```python
from build123d import *

# Parameters (mm, degrees)
BASESTEELANGLE_DEPTH = 150
TOEFILLET_R          = 10


with BuildPart() as part:
    # Sketch1 → BaseSteelAngle (new, symmetric)
    with BuildSketch(Plane.XY):
        with BuildLine():
            Line((0, 100), (0, 0))
            Line((0, 0), (100, 0))
            Line((100, 0), (100, 10))
            Line((100, 10), (22, 10))
            ThreePointArc((22, 10), (13.514718626, 13.514718626), (10, 22))
            Line((10, 22), (10, 100))
            Line((10, 100), (0, 100))
        make_face()
    extrude(amount=BASESTEELANGLE_DEPTH, both=True)

    # ToeFillet
    toefillet_edges = [part.edges().sort_by_distance(p)[0] for p in [
        (10, 100, 0),
        (100, 10, 0),
    ]]
    fillet(toefillet_edges, radius=TOEFILLET_R - 0.0001)  # a hair under: the kernel refuses the full size


solid = part.part
```
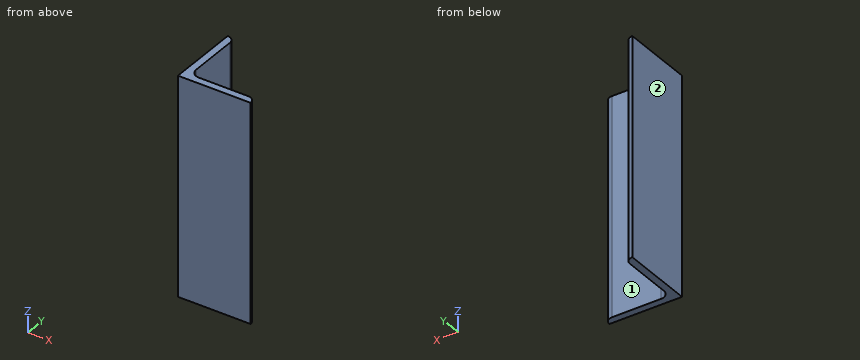
For this review, take the finished solid that the model builds, in its own axes (mm). Face numbers are marked on the shaded views. A direction names the side the tool comes from. Coordinates: 2 decimals unless noted, no trailing zeros. Loops run counter-clockwise (first coordinate to the right, second up) from the corner with the lowest first, then second, coordinate; pieces in that order, holes last. Notation, with made-up numbers: (3, 10.5) -> (47, 10.5) arc R9 ccw to (47, 21.5) -> close; hole circle Ø2 at (31.25, -36.75). An arc over 180 degrees is marked (long way). Return JSON: item names as keys, results as strings. Group by question number.
(1) Consider section B-B, the plane y = 49. Give the boundary of the cut face in (x, z).
(2) For pin 1 Ø3 at (y, z) = (43, 85.5) entering from +X; pin 2 Ø2 at (x, z) = (69, 40) entering from +Y, all flat-tipped, find the tip position at first contact; note any pin that passes through.
(3) To check wall thickness, follow L1, parallel to Y at x = 75.5, z = 86; L2, parallel to X at y = 94.5, z = -109. State the ranges of each line that lie inside material, in increasing order.
(4) Tool access review of the marked faces 1 and 2: name each direction out of +Z, -Z, +X, -X, +Y, -Y from which nothing blocks a thin tool from reaching the whole face with its end or side.
Results below:
{
 "1": {"outline": "(0, -150) -> (10, -150) -> (10, 150) -> (0, 150) -> close"},
 "2": {"pin 1": "stops at x = 10", "pin 2": "stops at y = 10"},
 "3": {"L1": "y = 0 to 10", "L2": "x = 0 to 8.93"},
 "4": {"face 1": "+Z, -Z, +X, +Y", "face 2": "+Z, -Z, -X, +Y, -Y"}
}
